```python
from build123d import *

# Parameters (mm, degrees)
ESQUISSE1_W      = 30
ESQUISSE1_H      = 60
ESQUISSE1_R      = 2.5
EXTRUSION1_DEPTH = 30
CONG_1_R         = 2


with BuildPart() as part:
    # Esquisse1 → Extrusion1 (new body)
    with BuildSketch(Plane.XY):
        with Locations((15, 30)):
            Rectangle(ESQUISSE1_W, ESQUISSE1_H)
        with Locations((10, 50)):
            Circle(ESQUISSE1_R, mode=Mode.SUBTRACT)
        with Locations((10, 10)):
            Circle(ESQUISSE1_R, mode=Mode.SUBTRACT)
    extrude(amount=EXTRUSION1_DEPTH)

    # Congé1
    cong_1_edges = [part.edges().sort_by_distance(p)[0] for p in [
        (30, 30, 30),
        (0, 30, 30),
        (30, 30, 0),
        (0, 30, 0),
    ]]
    fillet(cong_1_edges, radius=CONG_1_R)


solid = part.part
```
Input: part model. Units: mm. Frame: model coordinates. Round coordinates to 2 decimals unless told otherwise and drop trailing zeros. Loops run counter-clockwise (first coordinate to the right, second up) from the corner with the lowest first, then second, coordinate; pieces in that order, holes last. Notation, with made-up numbers: (82, 81.25) - (117, 81.25) arc R18 ccw to (117, 110.25) - close; hole circle Ø11 at (74.5, 16). An arc over 180 degrees is marked (long way). One line per item, written item: value. Start each with the question number.
(1) Draft query along Y for faces 1 (the cylindrical face through (0.57, 30.42, 0.6)), 2 (the cylindrical face through (9.46, 7.56, 14.79)), 3 (the flat face through (15, 60, 15)), 4 (the cylindrical face through (9.46, 47.56, 14.79)). Return one class per face: +Y half, -Y half, draft (parallel to the pull), parting line (faces both ways), or undercut.
(2) Ray query, line 1 (Y direction, x = 10, z = 21.5); line 2 (Y direction, x = 12, z = 26.75). Return the intervals inside material, ascending. Write a range as [from, to].
(3) Contact query for flat-ended pins moving along their axis: P1, Ø6.5, axis at x = 10, y = 10, coming from the +Z side; P2, Ø3, axis at x = 10, y = 50, coming from the +Z side. Output: stop coordinate, or through.
(4) Section B-B, the plane z = 25.25. Return loops of the section in (x, y), plus the area to 3 significant figures.
(5) Section A-A, the plane x = 10. Return loops of the section in (y, z), plus the area to 3 significant figures.
(6) Section C-C, the plane y = 10. Return loops of the section in (x, z).
Results below:
1. face 1: draft
1. face 2: undercut
1. face 3: +Y half
1. face 4: undercut
2. line 1: [0, 7.5], [12.5, 47.5], [52.5, 60]
2. line 2: [0, 8.5], [11.5, 48.5], [51.5, 60]
3. P1: z = 30
3. P2: through
4. outline: (0, 0) - (30, 0) - (30, 60) - (0, 60) - close; hole circle Ø5 at (10, 10); hole circle Ø5 at (10, 50)
4. area: 1,760 mm^2
5. outline: (0, 0) - (7.5, 0) - (7.5, 30) - (0, 30) - close; (12.5, 0) - (47.5, 0) - (47.5, 30) - (12.5, 30) - close; (52.5, 0) - (60, 0) - (60, 30) - (52.5, 30) - close
5. area: 1,500 mm^2
6. outline: (0, 2) arc R2 ccw to (2, 0) - (7.5, 0) - (7.5, 30) - (2, 30) arc R2 ccw to (0, 28) - close; (12.5, 0) - (28, 0) arc R2 ccw to (30, 2) - (30, 28) arc R2 ccw to (28, 30) - (12.5, 30) - close
